from build123d import *

# Parameters (mm, degrees)
SKETCH_1_W          = 8
SKETCH_1_H          = 4
EXTRUDE_1_DEPTH     = 3
CUT_EXTRUDE_1_DEPTH = 10
CUT_EXTRUDE_2_DEPTH = 10
CUT_EXTRUDE_3_DEPTH = 10
SKETCH_5_W          = 0.28903002
SKETCH_5_H          = 2.650043114
EXTRUDE_2_DEPTH     = 2
SKETCH_6_R          = 1.074823955
EXTRUDE_3_DEPTH     = 0.7
SKETCH_8_R          = 1.07
EXTRUDE_4_DEPTH     = 0.7
SKETCH_13_W         = 0.51855386
SKETCH_13_H         = 0.433545031
SKETCH_13_W_2       = 0.442045914
EXTRUDE_5_DEPTH     = 3.5
SKETCH_14_W         = 0.22952384
SKETCH_14_H         = 0.414585327
EXTRUDE_6_DEPTH     = 3.5


with BuildPart() as part:
    # 草图1 → 凸台-拉伸1 (new body)
    with BuildSketch(Plane(origin=(0, 0, 0), x_dir=(1, 0, 0), z_dir=(0, 1, 0))):
        Rectangle(SKETCH_1_W, SKETCH_1_H)
    extrude(amount=EXTRUDE_1_DEPTH)

    # 草图2 → 切除-拉伸1 (cut)
    with BuildSketch(Plane.ZY.offset(4)):
        Polygon((-2, 2.325021557), (-1.325021557, 3), (-2, 3), align=None)
        Polygon((2, 2.325021557), (1.325021557, 3), (2, 3), align=None)
    extrude(amount=-CUT_EXTRUDE_1_DEPTH, mode=Mode.SUBTRACT)

    # 草图3 → 切除-拉伸2 (cut)
    with BuildSketch(Plane.XY.offset(2)):
        Polygon((-4, 2.325021557), (-3.325021557, 3), (-4, 3), align=None)
        Polygon((4, 2.325021557), (3.325021557, 3), (4, 3), align=None)
    extrude(amount=-CUT_EXTRUDE_2_DEPTH, mode=Mode.SUBTRACT)

    # 草图4 → 切除-拉伸3 (cut)
    with BuildSketch(Plane(origin=(0, 3, 0), x_dir=(1, 0, 0), z_dir=(0, 1, 0))):
        Polygon((-3.325021557, 1.325021557), (-2.650043113, 2), (-4, 2), (-4, 0.650043113), align=None)
        Polygon((-3.325021557, -1.325021557), (-2.650043113, -2), (-4, -2), (-4, -0.650043113), align=None)
    extrude(amount=-CUT_EXTRUDE_3_DEPTH, mode=Mode.SUBTRACT)

    # 草图5 → 凸台-拉伸2 (add)
    with BuildSketch(Plane(origin=(0, 3, 0), x_dir=(1, 0, 0), z_dir=(0, 1, 0))):
        with Locations((-0.017001766, 0)):
            Rectangle(SKETCH_5_W, SKETCH_5_H)
    extrude(amount=EXTRUDE_2_DEPTH)

    # 草图6 → 凸台-拉伸3 (add)
    with BuildSketch(Plane(origin=(0, 3, 0), x_dir=(1, 0, 0), z_dir=(0, 1, 0))):
        with Locations(Location((-1.538659816, 0, 0), (0, 0, 90))):
            Circle(SKETCH_6_R)
    extrude(amount=EXTRUDE_3_DEPTH)

    # 草图7 → 旋转1 (revolve)
    with BuildSketch(Plane(origin=(0, 3.7, 0), x_dir=(1, 0, 0), z_dir=(0, 1, 0))):
        with BuildLine():
            Line((-0.463835861, 0), (-2.613483771, 0))
            ThreePointArc((-2.613483771, 0), (-1.538659816, -1.074823955), (-0.463835861, 0))
        make_face()
    revolve(axis=Axis((-0.463835861, 3.7, 0), (-1, 0, 0)))

    # 草图8 → 凸台-拉伸4 (add)
    with BuildSketch(Plane(origin=(0, 3, 0), x_dir=(1, 0, 0), z_dir=(0, 1, 0))):
        with Locations(Location((1.870194252, 0, 0), (0, 0, 90))):
            Circle(SKETCH_8_R)
    extrude(amount=EXTRUDE_4_DEPTH)

    # 草图12 → 旋转2 (revolve)
    with BuildSketch(Plane(origin=(0, 3.7, 0), x_dir=(1, 0, 0), z_dir=(0, 1, 0))):
        with BuildLine():
            Line((0.800194252, 0), (2.940194252, 0))
            ThreePointArc((2.940194252, 0), (1.870194252, -1.07), (0.800194252, 0))
        make_face()
    revolve(axis=Axis((0.800194252, 3.7, 0), (1, 0, 0)))

    # 草图13 → 凸台-拉伸5 (add)
    with BuildSketch(Plane.XZ):
        with Locations((-1.695926151, 0.884091829)):
            Rectangle(SKETCH_13_W, SKETCH_13_H)
        with Locations((-1.695926151, -1.198624497)):
            Rectangle(SKETCH_13_W, SKETCH_13_H)
        with Locations((2.371746347, 0.884091829)):
            Rectangle(SKETCH_13_W_2, SKETCH_13_H)
        with Locations((2.371746347, -1.198624497)):
            Rectangle(SKETCH_13_W_2, SKETCH_13_H)
    extrude(amount=EXTRUDE_5_DEPTH)

    # 草图14 → 凸台-拉伸6 (add)
    with BuildSketch(Plane.XZ):
        Polygon((0.187019425, 2), (0.187019425, 1.627919087), (0.416543265, 1.627919087), (0.416543265, 1.942451757), (0.416543265, 2), align=None)
        with Locations((0.301781345, -1.792707336)):
            Rectangle(SKETCH_14_W, SKETCH_14_H)
    extrude(amount=EXTRUDE_6_DEPTH)


solid = part.part
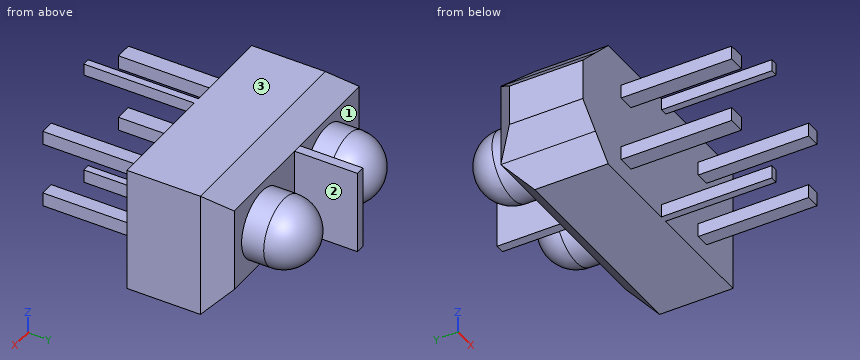
Read the model definition and answer for the solid it produces. Units are mm, in the model's axes. Face numbers are marked on the shaded views. A direction names the side the tool comes from. Round coordinates to 2 decimals unless told otherwise and drop trailing zeros. Write each loop counter-clockwise with the first axis right and the second up, starting at its lowest first coordinate (ties: lowest second). Pieces come first, ordered by that corner, then holes. Notation, with made-up numbers: (-27, 21.25) - (-15, 21.25) arc R23 cw to (-15, 57.25) - close; hole circle Ø8 at (86, -4). An arc over 180 degrees is marked (long way). Use a Markdown table: item, result.
(1) The part is cut by section C-C (y = 3.5). Write down the section's boundary in (x, z).
Reported:
| item | result |
|---|---|
| outline | circle Ø2.15 at (-1.54, 0); (-0.16, -1.33) - (0.13, -1.33) - (0.13, 1.33) - (-0.16, 1.33) - close; circle Ø2.14 at (1.87, 0) |
(2) The part is cut by section B-B (z = 0). Write down the section's boundary in (x, y).
Reported:
| item | result |
|---|---|
| outline | (-4, 0) - (4, 0) - (4, 2.33) - (3.33, 3) - (2.94, 3) - (2.94, 3.7) arc R1.07 ccw to (0.8, 3.7) - (0.8, 3) - (0.13, 3) - (0.13, 5) - (-0.16, 5) - (-0.16, 3) - (-0.46, 3) - (-0.46, 3.7) arc R1.07 ccw to (-2.61, 3.7) - (-2.61, 3) - (-3.33, 3) - (-4, 2.33) - close |
(3) The part is cut by section A-A (y = -0.5). Write down the section's boundary in (x, z), then the cut area to 3 significant figures.
Reported:
| item | result |
|---|---|
| outline | (-1.96, -1.42) - (-1.44, -1.42) - (-1.44, -0.98) - (-1.96, -0.98) - close; (-1.96, 0.67) - (-1.44, 0.67) - (-1.44, 1.1) - (-1.96, 1.1) - close; (0.19, -2) - (0.42, -2) - (0.42, -1.59) - (0.19, -1.59) - close; (0.19, 1.63) - (0.42, 1.63) - (0.42, 2) - (0.19, 2) - close; (2.15, -1.42) - (2.59, -1.42) - (2.59, -0.98) - (2.15, -0.98) - close; (2.15, 0.67) - (2.59, 0.67) - (2.59, 1.1) - (2.15, 1.1) - close |
| area | 1.01 mm2 |
(4) Straight lines are drawn through the part: line 1 along Z through (x, y) = (-1.75, -0.75); line 2 along Y through (x, z) = (1, 0.85); line 3 along X through (y, z) = (-3, -1.8). For each, find the intervals that lie inside material, in ascending order. Write a range as [from, to].
Reported:
| item | result |
|---|---|
| line 1 | [-1.42, -0.98], [0.67, 1.1] |
| line 2 | [0, 3] |
| line 3 | [0.19, 0.42] |
(5) Each of these flat-tipped pins is pushed along its axis until it touches: pin 1 Ø1.5 at (y, z) = (-1.5, 1) entering from +X; pin 2 Ø2 at (x, z) = (2, 0) entering from +Y; pin 3 Ø2 at (x, y) = (-0.5, 3.5) entering from +Z (3 decimals). Where does it stop, or does it pass through?
Reported:
| item | result |
|---|---|
| pin 1 | x = 2.59 |
| pin 2 | y = 4.77 |
| pin 3 | z = 1.825 |
(6) The part is cut by section D-D (x = 2.25). Write down the section's boundary in (y, z).
Reported:
| item | result |
|---|---|
| outline | (-3.5, -1.42) - (0, -1.42) - (0, -2) - (2.33, -2) - (3, -1.33) - (3, -1) - (3.7, -1) arc R1 ccw to (3.7, 1) - (3, 1) - (3, 1.33) - (2.33, 2) - (0, 2) - (0, 1.1) - (-3.5, 1.1) - (-3.5, 0.67) - (0, 0.67) - (0, -0.98) - (-3.5, -0.98) - close |
(7) Which of the six approach directions +Z, -Z, +X, -X, +Y, -Y give full straight-line access (tool end or side, diameter ignored) to the marked faces 1, 2 and 3?
Reported:
| item | result |
|---|---|
| face 1 | +Y |
| face 2 | +Z, -Z, +Y |
| face 3 | +Z, +X, -X, +Y, -Y |
